Design review of the part built by this model. Coordinates are the model's own, in mm. Face numbers are marked on the shaded views. A direction names the side the tool comes from. Round coordinates to 2 decimals unless told otherwise and drop trailing zeros. Loops run counter-clockwise (first coordinate to the right, second up) from the corner with the lowest first, then second, coordinate; pieces in that order, holes last. Notation, with made-up numbers: (39.5, 62) - (59.5, 62) arc R21 cw to (59.5, 72) - close; hole circle Ø3 at (70, -24.75). An arc over 180 degrees is marked (long way). Use one line per item in the form item = value. Start each with the question number.
(1) For pin 1 (6 mm diameter, centred on y = -12.5, z = -50, fed in from +X); pin 2 (2 mm diameter, centred on x = 11, y = 58.5, fed in from +Z); pin 3 (3 mm diameter, centred on x = 2.5, z = -52, fed in from -Y), all flat-tipped, find the tip position at first contact; note any pin that passes through.
(2) We need section C-C, the plane x = -46. Write out the cut boundary in (y, z), then the cut area to 3 significant figures.
(3) We need section A-A, the plane y = 0. Write out the cut boundary in (x, z), then the cut area to 3 significant figures.
(4) Machinability: for the marked faces 5, 6, 7 and 8, which of the approach directions +Z, -Z, +X, -X, +Y, -Y give a long, thin tool a straight path to every point of the face, cutting with its end or side? Answer none if there is none.
(5) Wall thickness on probe 1 along Y at (x, z) = (-37, 0); probe 2 along Z at (x, y) = (0, 41): over which ranges is each line inside the solid? List them lowest first. Write a range as [from, to].
(6) The part is to be moulded in two halves that separate along Y. For the marked faces 1, 2, 3 and 4, say which applies: released by +Y, released by -Y, zero draft, split by the parting line, or undercut.
(7) We need section D-D, the plane z = 54.5. Write out the cut boundary in (x, y), then the cut area to 3 significant figures.
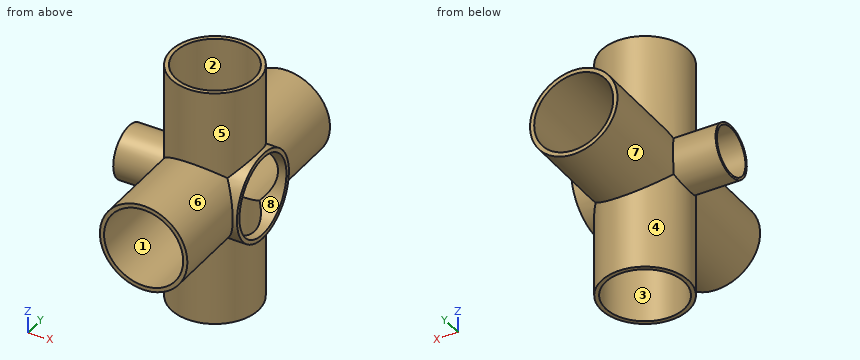
from build123d import *

# Parameters (mm, degrees)
SKETCH1_R               = 31.75
EXTRUDE3_DEPTH          = 87.122
EXTRUDE3_DEPTH_BACK     = 87.122
SKETCH4_R               = 31.75
EXTRUDE4_DEPTH          = 87.122
EXTRUDE4_DEPTH_BACK     = 87.122
SKETCH6_R               = 31.75
EXTRUDE5_DEPTH          = 34.798
SKETCH7_R               = 19.05
EXTRUDE6_DEPTH          = 62.484
SKETCH9_R               = 28.702
CUT_EXTRUDE1_DEPTH      = 88.1220001
CUT_EXTRUDE1_DEPTH_BACK = 88.1220001
SKETCH10_R              = 28.702
CUT_EXTRUDE2_DEPTH      = 88.1220001
CUT_EXTRUDE2_DEPTH_BACK = 88.1220001
SKETCH11_R              = 28.702
CUT_EXTRUDE3_DEPTH      = 35.798
SKETCH12_R              = 17.399
CUT_EXTRUDE4_DEPTH      = 63.4840001


with BuildPart() as part:
    # Sketch1 → Extrude3 (new body, two sides)
    with BuildSketch(Plane(origin=(0, 0, 0), x_dir=(1, 0, 0), z_dir=(0, 1, 0))) as extrude3_sk:
        Circle(SKETCH1_R)
    extrude(amount=EXTRUDE3_DEPTH)
    extrude(extrude3_sk.sketch, amount=-EXTRUDE3_DEPTH_BACK)

    # Sketch4 → Extrude4 (add, two sides)
    with BuildSketch(Plane.XY) as extrude4_sk:
        Circle(SKETCH4_R)
    extrude(amount=EXTRUDE4_DEPTH)
    extrude(extrude4_sk.sketch, amount=-EXTRUDE4_DEPTH_BACK)

    # Sketch6 → Extrude5 (add)
    with BuildSketch(Plane(origin=(0, 0, 0), x_dir=(0, 0, -1), z_dir=(1, 0, 0))):
        Circle(SKETCH6_R)
    extrude(amount=EXTRUDE5_DEPTH)

    # Sketch7 → Extrude6 (add)
    with BuildSketch(Plane(origin=(0, 0, 0), x_dir=(0, 0, -1), z_dir=(1, 0, 0))):
        Circle(SKETCH7_R)
    extrude(amount=-EXTRUDE6_DEPTH)

    # Sketch9 → Cut-Extrude1 (cut, two sides)
    with BuildSketch(Plane(origin=(0, 0, 0), x_dir=(1, 0, 0), z_dir=(0, 1, 0))) as cut_extrude1_sk:
        Circle(SKETCH9_R)
    extrude(amount=CUT_EXTRUDE1_DEPTH, mode=Mode.SUBTRACT)
    extrude(cut_extrude1_sk.sketch, amount=-CUT_EXTRUDE1_DEPTH_BACK, mode=Mode.SUBTRACT)

    # Sketch10 → Cut-Extrude2 (cut, two sides)
    with BuildSketch(Plane.XY) as cut_extrude2_sk:
        Circle(SKETCH10_R)
    extrude(amount=CUT_EXTRUDE2_DEPTH, mode=Mode.SUBTRACT)
    extrude(cut_extrude2_sk.sketch, amount=-CUT_EXTRUDE2_DEPTH_BACK, mode=Mode.SUBTRACT)

    # Sketch11 → Cut-Extrude3 (cut, through all)
    with BuildSketch(Plane(origin=(0, 0, 0), x_dir=(0, 0, -1), z_dir=(1, 0, 0))):
        Circle(SKETCH11_R)
    extrude(amount=CUT_EXTRUDE3_DEPTH, mode=Mode.SUBTRACT)

    # Sketch12 → Cut-Extrude4 (cut, through all)
    with BuildSketch(Plane(origin=(0, 0, 0), x_dir=(0, 0, -1), z_dir=(1, 0, 0))):
        Circle(SKETCH12_R)
    extrude(amount=-CUT_EXTRUDE4_DEPTH, mode=Mode.SUBTRACT)


solid = part.part
Data:
q1.pin_1 = 30.3
q1.pin_2 = 30.13
q1.pin_3 = -31.73
q2.outline = circle Ø38.1 at (0, 0); hole circle Ø34.8 at (0, 0)
q2.area = 189 mm^2
q3.outline = (-62.48, -19.05) - (-31.75, -19.05) - (-31.75, -87.12) - (-28.7, -87.12) - (-28.7, -17.4) - (-62.48, -17.4) - close; (-62.48, 17.4) - (-28.7, 17.4) - (-28.7, 87.12) - (-31.75, 87.12) - (-31.75, 19.05) - (-62.48, 19.05) - close; (28.7, -87.12) - (31.75, -87.12) - (31.75, -31.75) - (34.8, -31.75) - (34.8, -28.7) - (28.7, -28.7) - close; (28.7, 28.7) - (34.8, 28.7) - (34.8, 31.75) - (31.75, 31.75) - (31.75, 87.12) - (28.7, 87.12) - close
q3.area = 901 mm^2
q4.face_5 = +Z
q4.face_6 = -Y
q4.face_7 = +Y
q4.face_8 = +X
q5.probe_1 = [-19.05, -17.4], [17.4, 19.05]
q5.probe_2 = [-31.75, -28.7], [28.7, 31.75]
q6.face_1 = zero draft
q6.face_2 = undercut
q6.face_3 = undercut
q6.face_4 = split by the parting line
q7.outline = circle Ø63.5 at (0, 0); hole circle Ø57.4 at (0, 0)
q7.area = 579 mm^2
